from build123d import *

# Parameters (mm, degrees)
SKETCH1_W           = 22.86
SKETCH1_H           = 35.56
BOSS_EXTRUDE1_DEPTH = 1.6129
FILLET1_R           = 2.54
SKETCH2_W           = 8.5
SKETCH2_H           = 8.5
BOSS_EXTRUDE2_DEPTH = 5
CUT_EXTRUDE1_REACH  = 3.613
SKETCH3_R           = 1.5875
SKETCH4_R           = 2.54
CUT_EXTRUDE2_DEPTH  = 1.27


with BuildPart() as part:
    # Sketch1 → Boss-Extrude1 (new body)
    with BuildSketch(Plane.XY):
        Rectangle(SKETCH1_W, SKETCH1_H)
    extrude(amount=BOSS_EXTRUDE1_DEPTH)

    # Fillet1
    fillet1_edges = [part.edges().sort_by_distance(p)[0] for p in [
        (-11.43, 17.78, 0.80645),
        (11.43, 17.78, 0.80645),
    ]]
    fillet(fillet1_edges, radius=FILLET1_R)

    # Sketch2 → Boss-Extrude2 (add)
    with BuildSketch(Plane.XY.offset(1.6129)):
        with Locations((0, 11.625)):
            Rectangle(SKETCH2_W, SKETCH2_H)
    extrude(amount=BOSS_EXTRUDE2_DEPTH)

    # Sketch3 → Cut-Extrude1 (cut, up to next)
    with BuildSketch(Plane.XY.offset(1.6129), mode=Mode.PRIVATE) as cut_extrude1_sk1:
        with Locations((-8.89, 15.24)):
            Circle(SKETCH3_R)
    cut_extrude1_tool1 = extrude(cut_extrude1_sk1.sketch, amount=-CUT_EXTRUDE1_REACH, mode=Mode.PRIVATE) & part.part
    add(cut_extrude1_tool1.solids().sort_by_distance((-8.89, 15.24, 1.6129))[0], mode=Mode.SUBTRACT)
    # Sketch3 → Cut-Extrude1 (cut, up to next)
    with BuildSketch(Plane.XY.offset(1.6129), mode=Mode.PRIVATE) as cut_extrude1_sk2:
        with Locations((8.89, 15.24)):
            Circle(SKETCH3_R)
    cut_extrude1_tool2 = extrude(cut_extrude1_sk2.sketch, amount=-CUT_EXTRUDE1_REACH, mode=Mode.PRIVATE) & part.part
    add(cut_extrude1_tool2.solids().sort_by_distance((8.89, 15.24, 1.6129))[0], mode=Mode.SUBTRACT)

    # Sketch4 → Cut-Extrude2 (cut)
    with BuildSketch(Plane.XY.offset(6.6129)):
        with Locations((0, 11.625)):
            Circle(SKETCH4_R)
    extrude(amount=-CUT_EXTRUDE2_DEPTH, mode=Mode.SUBTRACT)


solid = part.part
Could you check a few things on this model? Use its own coordinates, in mm. A direction names the side the tool comes from. Round coordinates to 2 decimals unless told otherwise and drop trailing zeros. Order: outer loops, then holes, each group sorted by start corner. A loop starts at its lowest first (then second) coordinate and runs counter-clockwise, first axis right, second up. Notation, with made-up numbers: M 31,-6.75 L 51,-6.75 A23 cw 51,26.25 Z; hole C -6.5,-34 d11. An arc over 180 degrees is marked long. One line per item, written item: value.
(1) Imagine slicing it at D-D (z = 2.75). Write out the boundary of the cut face in (x, y) (3 decimals).
Ans:
outline: M -4.25,7.375 L 4.25,7.375 L 4.25,15.875 L -4.25,15.875 Z
(2) Imagine slicing it at A-A (z = 1). Write out the boundary of the cut face in (x, y) (1 decimal).
Ans:
outline: M -11.4,-17.8 L 11.4,-17.8 L 11.4,15.2 A2.5 ccw 8.9,17.8 L -8.9,17.8 A2.5 ccw -11.4,15.2 Z; hole C -8.9,15.2 d3.2; hole C 8.9,15.2 d3.2
(3) Imagine slicing it at B-B (x = 0). Write out the boundary of the cut face in (y, z) (3 decimals).
Ans:
outline: M -17.78,0 L 17.78,0 L 17.78,1.613 L 15.875,1.613 L 15.875,6.613 L 14.165,6.613 L 14.165,5.343 L 9.085,5.343 L 9.085,6.613 L 7.375,6.613 L 7.375,1.613 L -17.78,1.613 Z
(4) I'm going to push flat-ended pins straight in: P1, Ø12, axis at x = 2, y = -5.5, coming from the +Z side; P2, Ø3.5, axis at x = -8.89, y = 15.24, coming from the -Z side; P3, Ø4.5, axis at x = 0, y = 11.625, coming from the +Z side. Where does each tip first touch, or does it pass through?
Ans:
P1: stops at z = 1.61
P2: stops at z = 0
P3: stops at z = 5.34
(5) I need wall thicknesses on line 1 along Y through (x, z) = (0, 5.95) (3 decimals); line 2 along Y through (x, z) = (8.89, 0.85); line 3 along Z through (x, y) = (8.75, 0). Which ranges of each line are inside material? Lowest first, please. Write a range as from..to.
Ans:
line 1: y = 7.375..9.085, 14.165..15.875
line 2: y = -17.78..13.65, 16.83..17.78
line 3: z = 0..1.61
(6) If we mould it in two halves opening along Y, with no side actions, what happens to faces 4 (the flat face through (0, 17.78, 1)), 5 (the cylindrical face through (9.62, 13.83, 0.82)), 6 (the flat face through (0, 7.375, 4))? For each: released by +Y, released by -Y, zero draft, split by the parting line, or undercut.
Ans:
face 4: released by +Y
face 5: undercut
face 6: released by -Y
(7) Which directions (+Z, -Z, +X, -X, +Y, -Y) give clear straight access to the entire face, cutting with the end or side of a thin tool? Please do faces 1 (the flat face through (4.25, 12, 4)), 2 (the cylindrical face through (-0.551, 9.145, 5.987)), 3 (the flat face through (-4.25, 12, 4)).
Ans:
face 1: +Z, +X, +Y, -Y
face 2: +Z
face 3: +Z, -X, +Y, -Y
(8) Imagine slicing it at C-C (y = 12.5). Write out the boundary of the cut face in (x, z).
Ans:
outline: M -11.43,0 L 11.43,0 L 11.43,1.61 L 4.25,1.61 L 4.25,6.61 L 2.38,6.61 L 2.38,5.34 L -2.38,5.34 L -2.38,6.61 L -4.25,6.61 L -4.25,1.61 L -11.43,1.61 Z
